Work out the finished part from the listing and answer in its coordinate system (mm). Coordinates: 2 decimals unless noted, no trailing zeros. Order: outer loops, then holes, each group sorted by start corner. A loop starts at its lowest first (then second) coordinate and runs counter-clockwise, first axis right, second up. Notation, with made-up numbers: M 12,38.25 L 19,38.25 A26 ccw 19,60.25 Z; hole C -32,43.25 d9. An arc over 180 degrees is marked long. Use a Markdown table: item, result. Add a question column.
from build123d import *

# Parameters (mm, degrees)
SKETCH2_W             = 28.575
SKETCH2_H             = 133.35
BOSS_EXTRUDE1_DEPTH   = 9.525
F_3_0MM_DOWEL_HOLE1_D = 3
LPATTERN1_COUNT       = 4
LPATTERN1_PITCH       = 41.275
SKETCH8_R             = 1.5
CUT_EXTRUDE2_DEPTH    = 137.709468399


with BuildPart() as part:
    # Sketch2 → Boss-Extrude1 (new body)
    with BuildSketch(Plane(origin=(0, 0, 0), x_dir=(1, 0, 0), z_dir=(0, 1, 0))):
        with Locations((14.2875, 66.675)):
            Rectangle(SKETCH2_W, SKETCH2_H)
    extrude(amount=BOSS_EXTRUDE1_DEPTH)

    # Ø3.0mm Dowel Hole1 (through all)
    with Locations(Plane(origin=(28.575, 0, 0), x_dir=(0, 0, -1), z_dir=(1, 0, 0))):
        with Locations((4.7625, 4.7625)):
            f_3_0mm_dowel_hole1 = Hole(F_3_0MM_DOWEL_HOLE1_D / 2)

    # LPattern1: Ø3.0mm Dowel Hole1 ×4
    with Locations(*[(0, 0, -i * LPATTERN1_PITCH) for i in range(1, LPATTERN1_COUNT)]):
        add(f_3_0mm_dowel_hole1, mode=Mode.SUBTRACT)

    # Sketch8 → Cut-Extrude2 (cut, through all)
    with BuildSketch(Plane.XZ):
        with Locations(Location((9.525, -31.75, 0), (0, 0, 270))):
            Circle(SKETCH8_R)
        with Locations(Location((9.525, -101.6, 0), (0, 0, 270))):
            Circle(SKETCH8_R)
        with Locations(Location((19.05, -101.6, 0), (0, 0, 270))):
            Circle(SKETCH8_R)
        with Locations(Location((19.05, -31.75, 0), (0, 0, 270))):
            Circle(SKETCH8_R)
    extrude(amount=-CUT_EXTRUDE2_DEPTH, mode=Mode.SUBTRACT)


solid = part.part
(1) A cutting plane is placed at A-A on z = -101.6. Write down the section's boundary in (x, y) (3 decimals), plus the area to 3 significant figures.
(2) A cutting plane is placed at B-B on x = 19.05. Count the separate pieces of the cut face and the enclosed holes in it, plus the area to 3 significant figures.
(3) The mould has two halves that part along Y. Classify faces 1 (the flat face through (14, 5, -133.35)), 2 (the cylindrical face through (14.09, 4.19, -44.65)), 3 (the flat face through (14, 9.525, -68)), 4 (the cylindrical face through (14.087, 3.85, -5.953)): pulls with the +Y half, pulls with the -Y half, needs draft (parallel to the pull), parting line crosses it, or undercut.
(4) Straight lines are drawn through the part: line 1 (X direction, y = 7, z = -31.75) (3 decimals); line 2 (Z direction, x = 19, y = 7.25); line 3 (Z direction, x = 7.25, y = 5). For each, find the intervals that lie inside material, in ascending order.
(5) Given P1, Ø3, axis at x = 23, y = 4.5, coming from the +Z side, flat-ended and moving along its own axis, determine where the tip first touches the part or whether it passes through.
From the geometry:
| question | item | result |
|---|---|---|
| 1 | outline | M 0,0 L 8.025,0 L 8.025,9.525 L 0,9.525 Z; M 11.025,0 L 17.55,0 L 17.55,9.525 L 11.025,9.525 Z; M 20.55,0 L 28.575,0 L 28.575,9.525 L 20.55,9.525 Z |
| 1 | area | 215 mm2 |
| 2 | separate pieces | 3 |
| 2 | enclosed holes | 4 |
| 2 | area | 1,180 mm2 |
| 3 | face 1 | needs draft |
| 3 | face 2 | undercut |
| 3 | face 3 | pulls with the +Y half |
| 3 | face 4 | undercut |
| 4 | line 1 | x = 0 to 8.025, 11.025 to 17.55, 20.55 to 28.575 |
| 4 | line 2 | z = -133.35 to -103.1, -100.1 to -33.25, -30.25 to 0 |
| 4 | line 3 | z = -133.35 to -130.07, -127.11 to -88.79, -85.83 to -47.52, -44.56 to -6.24, -3.28 to 0 |
| 5 | P1 | stops at z = 0 |
